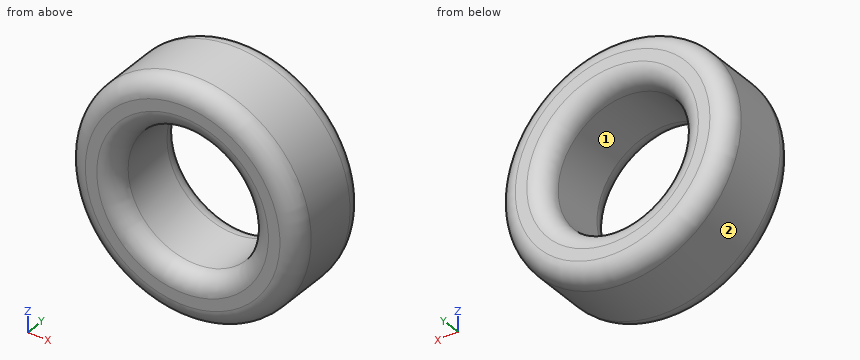
Autodesk Inventor part; units mm, degrees
ref_plane "YZ Plane" through (0, 0, 0) normal (1, 0, 0) x (0, 1, 0)
ref_plane "XZ Plane" through (0, 0, 0) normal (0, 1, 0) x (-1, 0, 0)
ref_plane "XY Plane" through (0, 0, 0) normal (0, 0, 1) x (1, 0, 0)
sketch "Sketch1" plane through (0, 0, 0) normal (0, 1, 0) x (-1, 0, 0)
  circle A0 centre (0, 0) radius 12.6074
  circle A1 centre (0, 0) radius 7.3543
extrude "Extrusion1" add sketch "Sketch1" along normal blind 10
fillet "Fillet1" radius 2 2 edges at (12.6074, 10, 0) (12.6074, 0, 0)
fillet "Fillet2" radius 2 2 edges at (7.3543, 10, 0) (7.3543, 0, 0)
Build history of the part. All positions in model axes, mm. Face numbers are marked on the shaded views. Coordinates: 2 decimals unless noted, no trailing zeros. Order: outer loops, then holes, each group sorted by start corner. A loop starts at its lowest first (then second) coordinate and runs counter-clockwise, first axis right, second up. Notation, with made-up numbers: (17.25, 81) -> (48.25, 81) arc R18 ccw to (48.25, 111) -> close; hole circle Ø6 at (-28, 58). An arc over 180 degrees is marked (long way). One line per item, written item: value.
(1) Slice it at B-B, the plane x = 0. List the corners of the cut face in (y, z), plus the area to 3 significant figures.
Checked values:
outline: (0, -10.61) arc R2 ccw to (2, -12.61) -> (8, -12.61) arc R2 ccw to (10, -10.61) -> (10, -9.35) arc R2 ccw to (8, -7.35) -> (2, -7.35) arc R2 ccw to (0, -9.35) -> close; (0, 9.35) arc R2 ccw to (2, 7.35) -> (8, 7.35) arc R2 ccw to (10, 9.35) -> (10, 10.61) arc R2 ccw to (8, 12.61) -> (2, 12.61) arc R2 ccw to (0, 10.61) -> close
area: 98.2 mm2
(2) Mould opens along Z. For the marked faces 1 and 2 say: pulls with the +Z half, pulls with the -Z half, needs draft (parallel to the pull), parting line crosses it, or undercut.
Checked values:
face 1: undercut
face 2: parting line crosses it
(3) Slice it at A-A, the plane z = 0. List the corners of the cut face in (x, y).
Checked values:
outline: (-12.61, 2) arc R2 ccw to (-10.61, 0) -> (-9.35, 0) arc R2 ccw to (-7.35, 2) -> (-7.35, 8) arc R2 ccw to (-9.35, 10) -> (-10.61, 10) arc R2 ccw to (-12.61, 8) -> close; (7.35, 2) arc R2 ccw to (9.35, 0) -> (10.61, 0) arc R2 ccw to (12.61, 2) -> (12.61, 8) arc R2 ccw to (10.61, 10) -> (9.35, 10) arc R2 ccw to (7.35, 8) -> close
(4) Slice it at C-C, the plane y = 5.5. List the corners of the cut face in (x, z), plus the area to 3 significant figures.
Checked values:
outline: circle Ø25.21 at (0, 0); hole circle Ø14.71 at (0, 0)
area: 329 mm2
(5) Slice it at D-D, the plane y = 1. List the corners of the cut face in (x, z), plus the area to 3 significant figures.
Checked values:
outline: circle Ø24.68 at (0, 0); hole circle Ø15.24 at (0, 0)
area: 296 mm2
(6) Drop flat-ended pins along their axis: pin 1 Ø6 at (x, y) = (-5.5, 6.5) entering from +Z; pin 2 Ø12 at (x, z) = (-0.5, -2.5) entering from -Y; pin 3 Ø4 at (x, y) = (10, 6) entering from +Z; pin 4 Ø6 at (x, y) = (1, 3.5) entering from +Z. Give the stop position or say it passes through.
Checked values:
pin 1: z = 12.36
pin 2: y = 0.17
pin 3: z = 9.74
pin 4: z = 12.61
(7) Probe line 1 (Z direction, x = 0, y = 5); line 2 (X direction, y = 8.5, z = 6.5); line 3 (Z direction, x = 4, y = 7.75). List the from-to ranges inside material, lowest first. Write a range as [from, to].
Checked values:
line 1: [-12.61, -7.35], [7.35, 12.61]
line 2: [-10.73, -3.57], [3.57, 10.73]
line 3: [-11.96, -6.17], [6.17, 11.96]
